Design review of the part shown in the three views and the two pictorial views. Dimensions are in mm from the part's minimum x, y and z. A direction names the side the tool comes from. Give positions to 0.01 mm unless a question says otherwise; leave off trailing zeros. Write each loop counter-clockwise with the first axis right and the second up, starting at its lowest first coordinate (ties: lowest second). Pieces come first, ordered by that corner, then holes. Notation, with made-up numbers: (-11.75, 55) -> (-6.75, 55) arc R12 ccw to (-6.75, 63) -> close; hole circle Ø5 at (-25, 40.25). An arc over 180 degrees is marked (long way). Use CSV: the item, a comma, the result in double quotes.
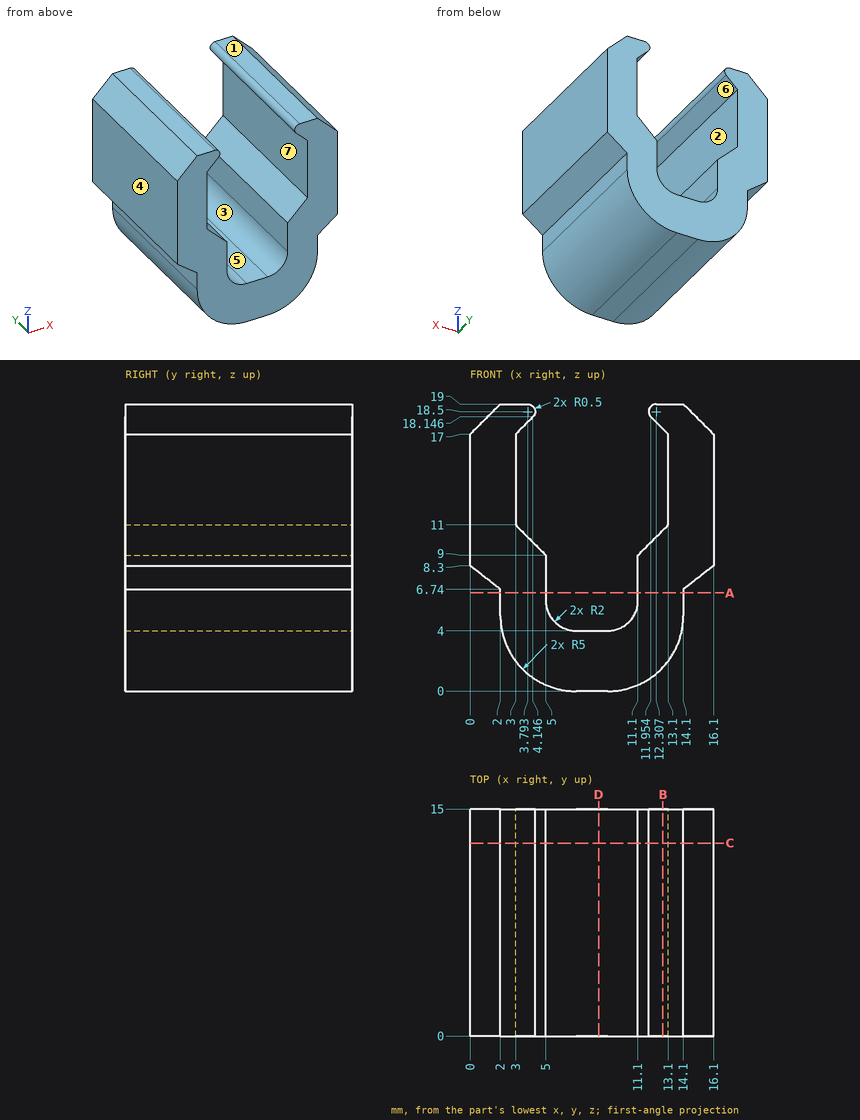
Q1. The part is to be moulded in two halves that separate along Z. For the marked faces 4, 5, 6 and 7, say which applies: pulls with the +Z half, pulls with the -Z half, needs draft (parallel to the pull), parting line crosses it, or undercut.
Derived:
face 4,"needs draft"
face 5,"pulls with the +Z half"
face 6,"undercut"
face 7,"undercut"
Q2. Consider section A-A (z = 6.5). Write out the cut boundary in (x, y).
Derived:
outline,"(2, 0) -> (5, 0) -> (5, 15) -> (2, 15) -> close; (11.1, 0) -> (14.1, 0) -> (14.1, 15) -> (11.1, 15) -> close"
Q3. Consider section D-D (x = 8.5). Write out the cut boundary in (y, z), then the cut area to 3 significant figures.
Derived:
outline,"(0, 0) -> (15, 0) -> (15, 4) -> (0, 4) -> close"
area,"60.0 mm2"
Q4. Machinability: for the marked faces 1, 2 and 3, which of the approach directions +Z, -Z, +X, -X, +Y, -Y give a long, thin tool a straight path to every point of the face, cutting with its end or side? Answer none if there is none.
Derived:
face 1,"+Z, +X, -X, +Y, -Y"
face 2,"+Y, -Y"
face 3,"+Z, +Y, -Y"
Q5. Insertion check: pin 1 (1.9 mm diameter, centred on y = 8, z = 6, fed in from +X); pin 2 (1.1 mm diameter, centred on x = 8, y = 9, fed in from +Z); pin 3 (1.5 mm diameter, centred on y = 4.5, z = 7.5, fed in from -X) (1 decimal). Each pin has a flat end and moves straight along its axis. Give the tip position at first contact, or say it passes through.
Derived:
pin 1,"stops at x = 14.37"
pin 2,"stops at z = 4"
pin 3,"stops at x = 0.1"
Q6. Consider section B-B (x = 12.75). Write out the cut boundary in (y, z), then the cut area to 3 significant figures.
Derived:
outline,"(0, 1.58) -> (15, 1.58) -> (15, 10.65) -> (0, 10.65) -> close; (0, 17.35) -> (15, 17.35) -> (15, 19) -> (0, 19) -> close"
area,"161 mm2"
Q7. Consider section C-C (y = 12.75). Write out the cut boundary in (x, z).
Derived:
outline,"(0, 8.3) -> (2, 6.74) -> (2, 5) arc R5 ccw to (7, 0) -> (9.1, 0) arc R5 ccw to (14.1, 5) -> (14.1, 6.74) -> (16.1, 8.3) -> (16.1, 17) -> (14.1, 19) -> (12.31, 19) arc R0.5 ccw to (11.95, 18.15) -> (13.1, 17) -> (13.1, 11) -> (11.1, 9) -> (11.1, 6) arc R2 cw to (9.1, 4) -> (7, 4) arc R2 cw to (5, 6) -> (5, 9) -> (3, 11) -> (3, 17) -> (4.15, 18.15) arc R0.5 ccw to (3.79, 19) -> (2, 19) -> (0, 17) -> close"
Q8. To check wall thickness, follow probe 1 along X at (y, z) = (11.5, 16); probe 2 along X at (y, z) = (13, 8.5); probe 3 along Z at (x, y) = (3.75, 13.5). State the ranges of each line that lie inside material, in increasing order.
Derived:
probe 1,"x = 0 to 3, 13.1 to 16.1"
probe 2,"x = 0 to 5, 11.1 to 16.1"
probe 3,"z = 1.2 to 10.25, 17.75 to 19"
